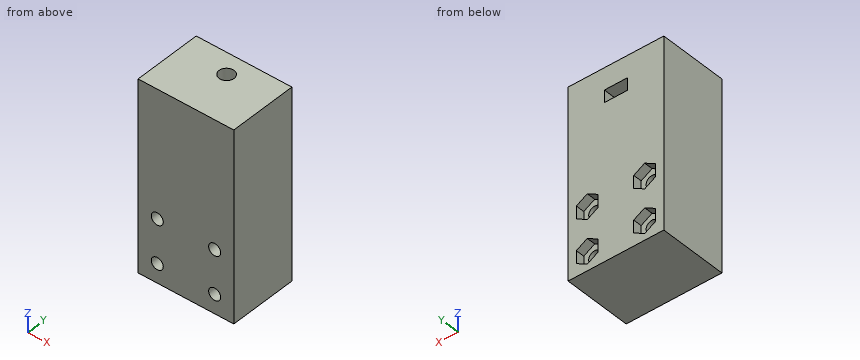
```python
from build123d import *

# Parameters (mm, degrees)
SKETCH_W        = 25
SKETCH_H        = 69.5
PAD_DEPTH       = 17.5
POCKET_DEPTH    = 4.5
SKETCH003_R     = 2.75
HOLE001_DEPTH   = 12
SKETCH004_R     = 2.2
HOLE_DEPTH      = 25.001
POCKET001_DEPTH = 3.2


with BuildPart() as part:
    # Sketch → Pad (new body, symmetric)
    with BuildSketch(Plane.YZ):
        with Locations((42.5, -44.75)):
            Rectangle(SKETCH_W, SKETCH_H)
    extrude(amount=PAD_DEPTH, both=True)

    # Sketch002 → Pocket (cut)
    with BuildSketch(Plane(origin=(0, 0, -18), x_dir=(0, -1, 0), z_dir=(0, 0, 1))):
        Polygon((-55, -4.25), (-55, 4.25), (-45.046262, 4.25), (-42.592523, 0), (-45.046262, -4.25), align=None)
    extrude(amount=-POCKET_DEPTH, mode=Mode.SUBTRACT)

    # Sketch003 (on Face2 of Pocket) → Hole001 (cut)
    with BuildSketch(Plane(origin=(0, 0, -10), x_dir=(0, -1, 0), z_dir=(0, 0, 1))):
        with Locations((-47.5, 0)):
            Circle(SKETCH003_R)
    extrude(amount=-HOLE001_DEPTH, mode=Mode.SUBTRACT)

    # Sketch004 (on Face6 of Hole001) → Hole (cut, through all)
    with BuildSketch(Plane.ZX.offset(55)):
        with Locations((-72.5, 10.5)):
            Circle(SKETCH004_R)
        with Locations((-56.5, 10.5)):
            Circle(SKETCH004_R)
        with Locations((-72.5, -10.5)):
            Circle(SKETCH004_R)
        with Locations((-56.5, -10.5)):
            Circle(SKETCH004_R)
    extrude(amount=-HOLE_DEPTH, mode=Mode.SUBTRACT)

    # Sketch005 (on Face10 of Hole) → Pocket001 (cut)
    with BuildSketch(Plane.ZX.offset(55)):
        Polygon((-70.190599, 14.5), (-74.809401, 14.5), (-77.118802, 10.5), (-74.809401, 6.5), (-70.190599, 6.5), (-67.881198, 10.5), align=None)
        Polygon((-51.881198, 10.5), (-54.190599, 14.5), (-58.809401, 14.5), (-61.118802, 10.5), (-58.809401, 6.5), (-54.190599, 6.5), align=None)
        Polygon((-51.881198, -10.5), (-54.190599, -6.5), (-58.809401, -6.5), (-61.118802, -10.5), (-58.809401, -14.5), (-54.190599, -14.5), align=None)
        Polygon((-70.190599, -6.5), (-74.809401, -6.5), (-77.118802, -10.5), (-74.809401, -14.5), (-70.190599, -14.5), (-67.881198, -10.5), align=None)
    extrude(amount=-POCKET001_DEPTH, mode=Mode.SUBTRACT)


solid = part.part
```
Verification items for the finished model (mm, model axes). Round coordinates to 2 decimals unless told otherwise and drop trailing zeros. Write each loop counter-clockwise with the first axis right and the second up, starting at its lowest first coordinate (ties: lowest second). Pieces come first, ordered by that corner, then holes. Notation, with made-up numbers: (-19.5, 38) -> (31.5, 38) arc R21 ccw to (31.5, 62) -> close; hole circle Ø6 at (58, -2). An arc over 180 degrees is marked (long way). Write each question's results on one line, items separated by ' | '. Start each with the question number.
1. Cross-section at C-C (x = 11.5). Enter the section's corners in (y, z).
2. Cross-section at A-A (z = -72.5). Enter the section's corners in (x, y), then the cut area to 3 significant figures.
3. Material ranges on probe 1 along X at (y, z) = (45.75, -56.5); probe 2 along Z at (x, y) = (4, 51.5); probe 3 along X at (y, z) = (47.5, -13.75), recorded low to high. Write a range as from..to.
4. Cross-section at D-D (y = 47.5). Enter the section's corners in (x, z).
5. Cross-section at B-B (y = 32). Enter the section's corners in (x, z), then the cut area to 3 significant figures.
6. Depth check by flat-ended pin: P1, Ø2.5, axis at x = -12, z = -74, coming from the +Y side. Enter the tip coordinate at first touch or a pass-through.
Solutions:
1) outline: (30, -79.5) -> (55, -79.5) -> (55, -76.54) -> (51.8, -76.54) -> (51.8, -74.46) -> (30, -74.46) -> close; (30, -70.54) -> (51.8, -70.54) -> (51.8, -68.46) -> (55, -68.46) -> (55, -60.54) -> (51.8, -60.54) -> (51.8, -58.46) -> (30, -58.46) -> close; (30, -54.54) -> (51.8, -54.54) -> (51.8, -52.46) -> (55, -52.46) -> (55, -10) -> (30, -10) -> close
2) outline: (-17.5, 30) -> (-12.7, 30) -> (-12.7, 51.8) -> (-14.5, 51.8) -> (-14.5, 55) -> (-17.5, 55) -> close; (-8.3, 30) -> (8.3, 30) -> (8.3, 51.8) -> (6.5, 51.8) -> (6.5, 55) -> (-6.5, 55) -> (-6.5, 51.8) -> (-8.3, 51.8) -> close; (12.7, 30) -> (17.5, 30) -> (17.5, 55) -> (14.5, 55) -> (14.5, 51.8) -> (12.7, 51.8) -> close | area: 632 mm2
3) probe 1: x = -17.5..-12.7, -8.3..8.3, 12.7..17.5 | probe 2: z = -79.5..-22.5, -18..-10 | probe 3: x = -17.5..-2.75, 2.75..17.5
4) outline: (-17.5, -79.5) -> (17.5, -79.5) -> (17.5, -10) -> (2.75, -10) -> (2.75, -18) -> (4.25, -18) -> (4.25, -22.5) -> (-4.25, -22.5) -> (-4.25, -18) -> (-2.75, -18) -> (-2.75, -10) -> (-17.5, -10) -> close; hole circle Ø4.4 at (-10.5, -72.5); hole circle Ø4.4 at (-10.5, -56.5); hole circle Ø4.4 at (10.5, -72.5); hole circle Ø4.4 at (10.5, -56.5)
5) outline: (-17.5, -79.5) -> (17.5, -79.5) -> (17.5, -10) -> (-17.5, -10) -> close; hole circle Ø4.4 at (-10.5, -72.5); hole circle Ø4.4 at (-10.5, -56.5); hole circle Ø4.4 at (10.5, -72.5); hole circle Ø4.4 at (10.5, -56.5) | area: 2,370 mm2
6) P1: stops at y = 51.8
